```python
from build123d import *

# Parameters (mm, degrees)
BOX001_W            = 10
BOX001_H            = 20
BOX001_DEPTH        = 10
BOX_W               = 10
BOX_H               = 30
BOX_DEPTH           = 8
CYLINDER_R          = 15
CYLINDER_DEPTH      = 30
CYLINDER_ROLL_ANGLE = 90


with BuildPart() as flat_top:
    # Box001 → Box001 (new body)
    with BuildSketch(Plane.XY.offset(7)):
        with Locations((5, 10)):
            Rectangle(BOX001_W, BOX001_H)
    extrude(amount=BOX001_DEPTH)


with BuildPart() as pin:
    # Box → Box (new body)
    with BuildSketch(Plane.XY):
        with Locations((5, 15)):
            Rectangle(BOX_W, BOX_H)
    extrude(amount=BOX_DEPTH)


with BuildPart() as cut:
    # Cylinder → Cylinder (new body)
    with BuildSketch(Plane.XY):
        Circle(CYLINDER_R)
    extrude(amount=CYLINDER_DEPTH)


with BuildPart() as cut_1:
    # Cylinder roll: moved
    add(cut.part.rotate(Axis((0, 0, 0), (1, 0, 0)), CYLINDER_ROLL_ANGLE))


with BuildPart() as cut_2:
    # Cylinder placement: moved
    add(cut_1.part.moved(Location((5, 25, -7))))

    # Common: intersect pin
    add(pin.part, mode=Mode.INTERSECT)

    # Cut: cut flat_top
    add(flat_top.part, mode=Mode.SUBTRACT)


solid = cut_2.part
```
Can you work these out from the model? Positions are in its coordinate system, mm. A direction names the side the tool comes from. Give positions to 0.01 mm unless a question says otherwise; leave off trailing zeros. Write each loop counter-clockwise with the first axis right and the second up, starting at its lowest first coordinate (ties: lowest second). Pieces come first, ordered by that corner, then holes. Notation, with made-up numbers: (81, 1.25) -> (128, 1.25) arc R7 cw to (128, 10.25) -> close; hole circle Ø9 at (44, 61.5). An arc over 180 degrees is marked (long way). One line per item, written item: value.
Q1. For P1, Ø6, axis at x = 6.5, y = 21.5, coming from the +Z side; P2, Ø0.8, axis at x = 3, z = 7.5, coming from the -Y side; P3, Ø3, axis at x = 4.5, y = 13.5, coming from the +Z side, each with a flat end and sliding along its axis, tell me the tip position at first contact or that it passes through.
Results found:
P1: stops at z = 8
P2: stops at y = 20
P3: stops at z = 7
Q2. Imagine slicing it at B-B on y = 2.25. Please give me the cut outline in (x, z).
Results found:
outline: (0, 0) -> (10, 0) -> (10, 7) -> (0, 7) -> close
Q3. Which directions (+Z, -Z, +X, -X, +Y, -Y) give clear straight access to the entire face, cutting with the end or side of a thin tool? Please do faces 1 (the face through (5, 25, 4)), 2 (the face through (4.9, 20, 7.4)).
Results found:
face 1: +Z, -Z, +X, -X, +Y
face 2: +Z, +X, -X, -Y
Q4. Imagine slicing it at C-C on x = 1.25. Please give me the cut outline in (y, z), and give its area (3 significant figures).
Results found:
outline: (0, 0) -> (25, 0) -> (25, 7.52) -> (20, 7.52) -> (20, 7) -> (0, 7) -> close
area: 178 mm^2
Q5. Please list where these lines run through material, in increasing order: line 1 (Z direction, x = 5.75, y = 16.25); line 2 (Z direction, x = 5, y = 22.5); line 3 (Y direction, x = 6.25, z = 7.75). Write a range as [from, to].
Results found:
line 1: z = [0, 7]
line 2: z = [0, 8]
line 3: y = [20, 25]
Q6. Imagine slicing it at A-A on x = 7. Please give me the cut outline in (y, z).
Results found:
outline: (0, 0) -> (25, 0) -> (25, 7.87) -> (20, 7.87) -> (20, 7) -> (0, 7) -> close
Q7. Imagine slicing it at D-D on y = 21.5. Please give me the cut outline in (x, z), and give its area (3 significant figures).
Results found:
outline: (0, 0) -> (10, 0) -> (10, 7.14) arc R15 ccw to (0, 7.14) -> close
area: 77.2 mm^2
